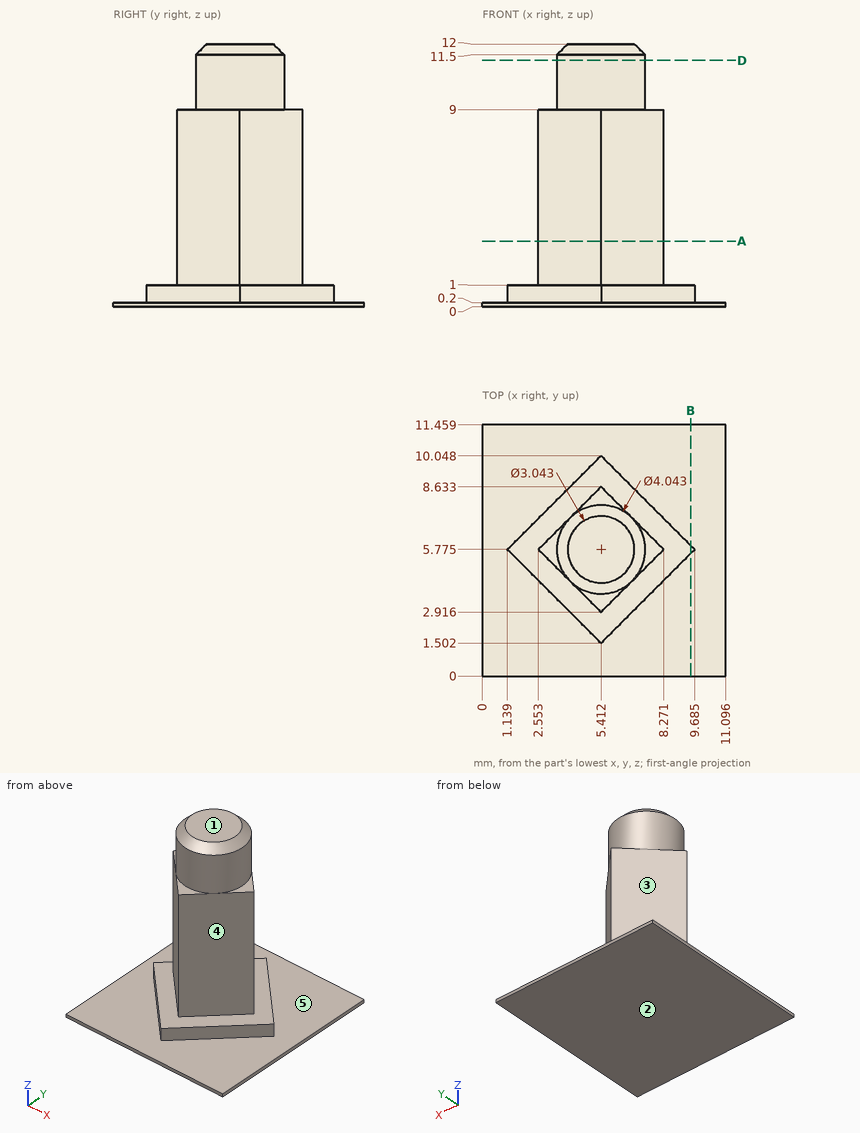
Could you check a few things on this drawing? It's one solid part, dimensions in mm from its lowest x, y, z. A direction names the side the tool comes from. Coordinates: 2 decimals unless noted, no trailing zeros. Write each loop counter-clockwise with the first axis right and the second up, starting at its lowest first coordinate (ties: lowest second). Pieces come first, ordered by that corner, then holes. Notation, with made-up numbers: (75.25, 19.25) - (88.25, 19.25) arc R7 ccw to (88.25, 28.25) - close; hole circle Ø3 at (20.25, 31). An arc over 180 degrees is marked (long way). Return JSON: item names as keys, results as strings. Group by question number.
Item 1: If we section it at D-D (z = 11.25): Write out the boundary of the cut face in (x, y) (1 decimal), then the cut area to 3 significant figures.
Item 2: If we section it at A-A (z = 3): Write out the boundary of the cut face in (x, y) (1 decimal).
Item 3: If we section it at B-B (x = 9.5): Write out the boundary of the cut face in (y, z).
Item 4: Which directions (+Z, -Z, +X, -X, +Y, -Y) give clear straight access to the entire face, cutting with the end or side of a thin tool? Please do the marked faces 1, 2, 3, 4 and 5.
Item 5: I'm going to push flat-ended pins straight in: pin 1 Ø5 at (y, z) = (2.5, 4.5) entering from -X; pin 2 Ø1.5 at (x, z) = (6.5, 8.5) entering from +Y (1 decimal); pin 3 Ø4 at (x, y) = (9, 8.5) entering from +Z; pin 4 Ø1.5 at (x, z) = (1.5, 3) entering from +Y. Where does each tip first touch, or does it pass through?
Item 6: Please list where these lines run through material, in increasing order: probe 1 along Z at (x, y) = (2.5, 9.5); probe 2 along Y at (x, z) = (6.25, 7.75) (1 decimal); probe 3 along X at (y, z) = (7.5, 2.25) (1 decimal).
Return value:
{
 "1": {"outline": "circle Ø4 at (5.4, 5.8)", "area": "12.8 mm^2"},
 "2": {"outline": "(2.6, 5.8) - (5.4, 2.9) - (8.3, 5.8) - (5.4, 8.6) - close"},
 "3": {"outline": "(0, 0) - (11.46, 0) - (11.46, 0.2) - (5.96, 0.2) - (5.96, 1) - (5.59, 1) - (5.59, 0.2) - (0, 0.2) - close"},
 "4": {"face 1": "+Z, +X, -X, +Y, -Y", "face 2": "-Z, +X, -X, +Y, -Y", "face 3": "+Z, -X, +Y", "face 4": "+Z, +X, -Y", "face 5": "+Z"},
 "5": {"pin 1": "stops at x = 3.33", "pin 2": "stops at y = 8.3", "pin 3": "stops at z = 1", "pin 4": "passes through"},
 "6": {"probe 1": "z = 0 to 0.2", "probe 2": "y = 3.8 to 7.8", "probe 3": "x = 4.3 to 6.5"}
}
